```python
from build123d import *

# Parameters (mm, degrees)
F1_DEPTH = 25.4
F3_DEPTH = 25.4
F5_DEPTH = 25.4
F7_DEPTH = 25.4


with BuildPart() as f1:
    # F0 (on Front) → F1 (new body)
    with BuildSketch(Plane.XZ):
        Polygon((-25.4, 12.7), (-25.4, 0), (50.8, 0), (50.8, 12.7), (25.4, 12.7), (25.4, 44.45), (0, 44.45), (0, 12.7), align=None)
    extrude(amount=F1_DEPTH)

    # F2 (on face) → F3 (cut)
    with BuildSketch(Plane.YZ.offset(25.4)):
        with BuildLine():
            Line((-25.4, 28.575), (-25.4, 38.1))
            ThreePointArc((-25.4, 38.1), (-28.575, 28.575), (-25.4, 19.05))
            Line((-25.4, 19.05), (-25.4, 28.575))
        make_face()
        with BuildLine():
            ThreePointArc((3.175, 28.575), (2.3603473566, 33.5951157855), (0, 38.1))
            Line((0, 38.1), (0, 28.575))
            Line((0, 28.575), (0, 19.05))
            ThreePointArc((0, 19.05), (2.3603473566, 23.5548842145), (3.175, 28.575))
        make_face()
        with BuildLine():
            Line((0, 44.45), (-12.7, 44.45))
            ThreePointArc((-12.7, 44.45), (-5.6004841714, 42.7740316571), (0, 38.1))
            Line((0, 38.1), (0, 44.45))
        make_face()
        with BuildLine():
            ThreePointArc((-25.4, 38.1), (-19.7995158286, 42.7740316571), (-12.7, 44.45))
            Line((-12.7, 44.45), (-25.4, 44.45))
            Line((-25.4, 44.45), (-25.4, 38.1))
        make_face()
        with BuildLine():
            ThreePointArc((-6.3216395999, 28.575), (-8.1898181082, 33.0851818918), (-12.7, 34.9533604001))
            Line((-12.7, 34.9533604001), (-12.7, 28.575))
            Line((-12.7, 28.575), (-6.3216395999, 28.575))
        make_face()
        with BuildLine():
            Line((-12.7, 28.575), (-12.7, 34.9533604001))
            ThreePointArc((-12.7, 34.9533604001), (-17.2101818918, 33.0851818918), (-19.0783604001, 28.575))
            Line((-19.0783604001, 28.575), (-12.7, 28.575))
        make_face()
        with BuildLine():
            Line((-6.3216395999, 28.575), (-12.7, 28.575))
            Line((-12.7, 28.575), (-12.7, 22.1966395999))
            ThreePointArc((-12.7, 22.1966395999), (-8.1898181082, 24.0648181082), (-6.3216395999, 28.575))
        make_face()
        with BuildLine():
            Line((-12.7, 22.1966395999), (-12.7, 28.575))
            Line((-12.7, 28.575), (-19.0783604001, 28.575))
            ThreePointArc((-19.0783604001, 28.575), (-17.2101818918, 24.0648181082), (-12.7, 22.1966395999))
        make_face()
    extrude(amount=-F3_DEPTH, mode=Mode.SUBTRACT)

    # F4 (on face) → F5 (cut)
    with BuildSketch(Plane.XY.offset(12.7)):
        with BuildLine():
            Line((44.45, -12.7), (38.1, -12.7))
            Line((38.1, -12.7), (38.1, -19.05))
            ThreePointArc((38.1, -19.05), (42.5901280605, -17.1901280605), (44.45, -12.7))
        make_face()
        with BuildLine():
            ThreePointArc((44.45, -12.7), (42.5901280605, -8.2098719395), (38.1, -6.35))
            Line((38.1, -6.35), (38.1, -12.7))
            Line((38.1, -12.7), (44.45, -12.7))
        make_face()
        with BuildLine():
            Line((38.1, -12.7), (38.1, -6.35))
            ThreePointArc((38.1, -6.35), (33.6098719395, -8.2098719395), (31.75, -12.7))
            Line((31.75, -12.7), (38.1, -12.7))
        make_face()
        with BuildLine():
            Line((38.1, -19.05), (38.1, -12.7))
            Line((38.1, -12.7), (31.75, -12.7))
            ThreePointArc((31.75, -12.7), (33.6098719395, -17.1901280605), (38.1, -19.05))
        make_face()
        with BuildLine():
            Line((50.8, 0), (38.1, 0))
            ThreePointArc((38.1, 0), (47.0802561211, -3.7197438789), (50.8, -12.7))
            Line((50.8, -12.7), (50.8, 0))
        make_face()
        with BuildLine():
            Line((50.8, -25.4), (50.8, -12.7))
            ThreePointArc((50.8, -12.7), (47.0802561211, -21.6802561211), (38.1, -25.4))
            Line((38.1, -25.4), (50.8, -25.4))
        make_face()
    extrude(amount=-F5_DEPTH, mode=Mode.SUBTRACT)

    # F6 (on face) → F7 (cut)
    with BuildSketch(Plane.XY.offset(12.7)):
        with BuildLine():
            Line((-6.35, -12.7), (-12.7, -12.7))
            Line((-12.7, -12.7), (-12.7, -19.05))
            ThreePointArc((-12.7, -19.05), (-8.2098719395, -17.1901280605), (-6.35, -12.7))
        make_face()
        with BuildLine():
            Line((-12.7, -19.05), (-12.7, -12.7))
            Line((-12.7, -12.7), (-19.05, -12.7))
            ThreePointArc((-19.05, -12.7), (-17.1901280605, -17.1901280605), (-12.7, -19.05))
        make_face()
        with BuildLine():
            Line((-12.7, -12.7), (-12.7, -6.35))
            ThreePointArc((-12.7, -6.35), (-17.1901280605, -8.2098719395), (-19.05, -12.7))
            Line((-19.05, -12.7), (-12.7, -12.7))
        make_face()
        with BuildLine():
            ThreePointArc((-6.35, -12.7), (-8.2098719395, -8.2098719395), (-12.7, -6.35))
            Line((-12.7, -6.35), (-12.7, -12.7))
            Line((-12.7, -12.7), (-6.35, -12.7))
        make_face()
        with BuildLine():
            ThreePointArc((-12.7, -25.4), (-21.6802561211, -21.6802561211), (-25.4, -12.7))
            Line((-25.4, -12.7), (-25.4, -25.4))
            Line((-25.4, -25.4), (-12.7, -25.4))
        make_face()
        with BuildLine():
            ThreePointArc((-25.4, -12.7), (-21.6802561211, -3.7197438789), (-12.7, 0))
            Line((-12.7, 0), (-25.4, 0))
            Line((-25.4, 0), (-25.4, -12.7))
        make_face()
    extrude(amount=-F7_DEPTH, mode=Mode.SUBTRACT)


solid = f1.part
```
Could you check a few things on this model? Use its own coordinates, in mm. A direction names the side the tool comes from. Give positions to 0.01 mm unless a question says otherwise; leave off trailing zeros. Loops run counter-clockwise (first coordinate to the right, second up) from the corner with the lowest first, then second, coordinate; pieces in that order, holes last. Notation, with made-up numbers: (48, -2) - (68, -2) arc R32 ccw to (68, 33) - close; hole circle Ø3 at (9, 62). An arc over 180 degrees is marked (long way). Use one line per item in the form item = value.
1. I want a section at C-C (x = 32.5). Please give me the cut outline in (y, z), and give its area (3 significant figures).
Response values:
outline = (-25.4, 0) - (-15.69, 0) - (-15.69, 12.7) - (-25.4, 12.7) - close; (-9.71, 0) - (0, 0) - (0, 12.7) - (-9.71, 12.7) - close
area = 247 mm²
2. I'm going to push flat-ended pins straight in: pin 1 Ø2 at (x, y) = (38.5, -21) entering from +Z; pin 2 Ø7.5 at (y, z) = (-11, 33) entering from +X; pin 3 Ø6 at (y, z) = (-22.5, 9) entering from +X. Where does each tip first touch, or does it pass through?
Response values:
pin_1 = 12.7
pin_2 = 25.4
pin_3 = 48.83
3. On a 3-axis mill with a long thin cutter (end or side, diameter ignored), from which of +Z, -Z, +X, -X, +Y, -Y can I reach the whole of each face in a straight line? I mean faces 1 (the face through (25.4, -13, 21)), 2 (the face through (0, -13, 22)), 3 (the face through (12, -13, 0)). Say none if no direction works.
Response values:
face_1 = +Z, +X, +Y, -Y
face_2 = +Z, -X, +Y, -Y
face_3 = -Z, +X, -X, +Y, -Y
4. I need wall thicknesses on probe 1 along X at (y, z) = (-5, 35.5); probe 2 along Y at (x, z) = (10, 28.5); probe 3 along Z at (x, y) = (-16.5, -22). Which ranges of each line are inside material? Lowest first, please.
Response values:
probe_1 = 0 to 25.4
probe_2 = -25.4 to -19.08, -6.32 to 0
probe_3 = 0 to 12.7
5. I want a section at A-A (x = 10). Please give me the cut outline in (y, z) (3 decimals).
Response values:
outline = (-25.4, 0) - (0, 0) - (0, 38.1) arc R15.875 ccw to (-25.4, 38.1) - close; hole circle Ø12.757 at (-12.7, 28.575)
6. I want a section at B-B (z = 3.5). Please give me the cut outline in (x, y).
Response values:
outline = (-12.7, -25.4) - (38.1, -25.4) arc R12.7 ccw to (38.1, 0) - (-12.7, 0) arc R12.7 ccw to start; hole circle Ø12.7 at (-12.7, -12.7); hole circle Ø12.7 at (38.1, -12.7)
7. I want a section at D-D (y = -15). Please give me the cut outline in (x, z), and give its area (3 significant figures).
Response values:
outline = (-25.19, 0) - (-18.62, 0) - (-18.62, 12.7) - (-25.19, 12.7) - close; (-6.78, 0) - (32.18, 0) - (32.18, 12.7) - (25.4, 12.7) - (25.4, 22.63) - (0, 22.63) - (0, 12.7) - (-6.78, 12.7) - close; (0, 34.52) - (25.4, 34.52) - (25.4, 44.28) - (0, 44.28) - close; (44.02, 0) - (50.59, 0) - (50.59, 12.7) - (44.02, 12.7) - close
area = 1,160 mm²
